Design review of the part built by this model. Coordinates are the model's own, in mm. Face numbers are marked on the shaded views. A direction names the side the tool comes from. Round coordinates to 2 decimals unless told otherwise and drop trailing zeros. Loops run counter-clockwise (first coordinate to the right, second up) from the corner with the lowest first, then second, coordinate; pieces in that order, holes last. Notation, with made-up numbers: (-6, -25.5) - (40, -25.5) arc R23 ccw to (40, -4.5) - close; hole circle Ø1 at (-3, 30). An arc over 180 degrees is marked (long way). Return JSON: item names as keys, results as strings. Group by question number.
(1) Wall thickness on L1, parallel to Y at x = 12, z = 2.5; L2, parallel to Y at x = 0.7, z = 6; L3, parallel to Y at x = 10.75, z = -1.75: over which ranges is each line inside the solid? List them lowest first. Write a range as [from, to].
(2) We need section C-C, the plane z = -10. Write out the cut boundary in (x, y).
(3) For the marked faces 1, 2, 3 and 4, list the 3-axis set-ups (+Z, -Z, +X, -X, +Y, -Y) from which the entire face can be reached by the end or side of a thin tool; tool diameter is ignored.
(4) The part is to be moulded in two halves that separate along Y. For the marked faces 5, 6 and 7, say which applies: pulls with the +Y half, pulls with the -Y half, needs draft (parallel to the pull), parting line crosses it, or undercut.
(5) We need section D-D, the plane z = 6. Write out the cut boundary in (x, y).
(6) We need section A-A, the plane y = 1.5. Write out the cut boundary in (x, z).
(7) We need section B-B, the plane x = 10. Write out the cut boundary in (y, z).
(8) Clearance check with flat-ended pins moving along their axes: pin 1 (10 mm diameter, centred on x = 2.5, z = -1, fed in from -Y); pin 2 (3 mm diameter, centred on y = 2, z = 6, fed in from +X); pin 3 (5 mm diameter, centred on x = 8.5, y = -5, fed in from -Z); pin 4 (8.5 mm diameter, centred on x = 10, z = -10, fed in from -Y). State where each tip first meets the part, or that it passes through.
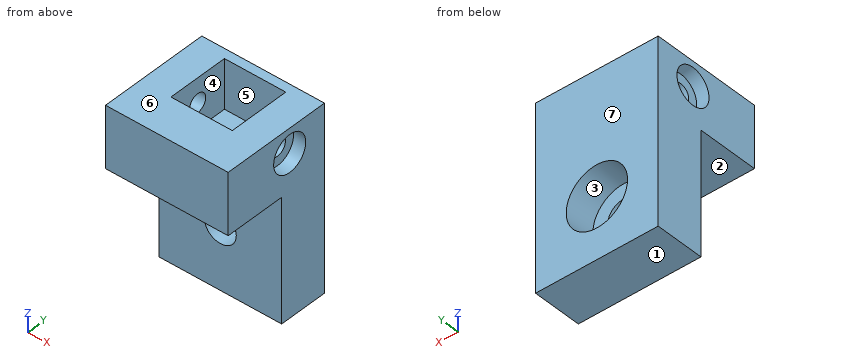
from build123d import *

# Parameters (mm, degrees)
SKETCH_1_W          = 20
SKETCH_1_H          = 20
EXTRUDE_1_DEPTH     = 8
EXTRUDE_2_DEPTH     = 20
SKETCH_3_W          = 4
SKETCH_3_H          = 13
EXTRUDE_3_DEPTH     = 20
CUT_EXTRUDE_1_DEPTH = 5
SKETCH_5_R          = 2.6
CUT_EXTRUDE_2_DEPTH = 13
EXTRUDE_4_DEPTH     = 20
SKETCH_9_W          = 20
SKETCH_9_H          = 13
SKETCH_9_W_2        = 10
SKETCH_9_H_2        = 10
EXTRUDE_5_DEPTH     = 26
SKETCH_10_W         = 10
SKETCH_10_H         = 10
CUT_EXTRUDE_3_DEPTH = 14
SKETCH_13_W         = 20
SKETCH_13_H         = 13
CUT_EXTRUDE_4_DEPTH = 20
SKETCH_14_W         = 5
SKETCH_14_H         = 5
CUT_EXTRUDE_5_DEPTH = 8
CUT_EXTRUDE_6_DEPTH = 20
SKETCH_16_R         = 3
CUT_EXTRUDE_7_DEPTH = 2
CUT_EXTRUDE_START   = -2
SKETCH_17_R         = 3
CUT_EXTRUDE_8_DEPTH = 2
SKETCH_18_W         = 20
SKETCH_18_H         = 4
CUT_EXTRUDE_9_DEPTH = 20
SKETCH_19_W         = 10
SKETCH_19_H         = 5
EXTRUDE_6_DEPTH     = 20


with BuildPart() as part:
    # 草图1 → 凸台-拉伸1 (new body)
    with BuildSketch(Plane(origin=(0, 0, 0), x_dir=(1, 0, 0), z_dir=(0, 1, 0))):
        with Locations((10, 10)):
            Rectangle(SKETCH_1_W, SKETCH_1_H)
    extrude(amount=EXTRUDE_1_DEPTH)

    # 草图2 → 凸台-拉伸2 (add)
    with BuildSketch(Plane.ZY):
        Polygon((-24, 0), (-24, -5), (-20, -5), (-20, 0), (-20, 8), (-24, 8), align=None)
    extrude(amount=-EXTRUDE_2_DEPTH)

    # 草图3 → 凸台-拉伸3 (add)
    with BuildSketch(Plane.ZY):
        with Locations((2, 1.5)):
            Rectangle(SKETCH_3_W, SKETCH_3_H)
    extrude(amount=-EXTRUDE_3_DEPTH)

    # 草图4 → 切除-拉伸1 (cut)
    with BuildSketch(Plane(origin=(0, 8, 0), x_dir=(1, 0, 0), z_dir=(0, 1, 0))):
        with BuildLine():
            ThreePointArc((15, 10), (10, 15), (5, 10))
            Line((5, 10), (15, 10))
        make_face()
        with BuildLine():
            Line((15, 10), (5, 10))
            ThreePointArc((5, 10), (10, 5), (15, 10))
        make_face()
        with BuildLine():
            ThreePointArc((15, 10), (10, 15), (5, 10))
            Line((5, 10), (15, 10))
        make_face()
        with BuildLine():
            Line((15, 10), (5, 10))
            ThreePointArc((5, 10), (10, 5), (15, 10))
        make_face()
    extrude(amount=-CUT_EXTRUDE_1_DEPTH, mode=Mode.SUBTRACT)

    # 草图5 → 切除-拉伸2 (cut)
    with BuildSketch(Plane(origin=(0, 8, 0), x_dir=(1, 0, 0), z_dir=(0, 1, 0))):
        with Locations(Location((10, 10, 0), (0, 0, 270))):
            Circle(SKETCH_5_R)
    extrude(amount=-CUT_EXTRUDE_2_DEPTH, mode=Mode.SUBTRACT)

    # 草图8 → 凸台-拉伸4 (add)
    with BuildSketch(Plane.XY.offset(4)):
        Polygon((10, 6.5), (15, 6.5), (15, 1.5), (15, -3.5), (10, -3.5), (5, -3.5), (5, 1.5), (5, 6.5), align=None)
    extrude(amount=EXTRUDE_4_DEPTH)

    # 草图9 → 凸台-拉伸5 (add)
    with BuildSketch(Plane.XY.offset(4)):
        with Locations((10, 1.5)):
            Rectangle(SKETCH_9_W, SKETCH_9_H)
        with Locations((10, 1.5)):
            Rectangle(SKETCH_9_W_2, SKETCH_9_H_2, mode=Mode.SUBTRACT)
    extrude(amount=EXTRUDE_5_DEPTH)

    # 草图10 → 切除-拉伸3 (cut)
    with BuildSketch(Plane.XY.offset(24)):
        with Locations((10, 1.5)):
            Rectangle(SKETCH_10_W, SKETCH_10_H)
    extrude(amount=-CUT_EXTRUDE_3_DEPTH, mode=Mode.SUBTRACT)

    # 草图13 → 切除-拉伸4 (cut)
    with BuildSketch(Plane.ZY):
        with Locations((20, 1.5)):
            Rectangle(SKETCH_13_W, SKETCH_13_H)
    extrude(amount=-CUT_EXTRUDE_4_DEPTH, mode=Mode.SUBTRACT)

    # 草图14 → 切除-拉伸5 (cut)
    with BuildSketch(Plane.XY.offset(10)):
        with Locations((7.5, 4)):
            Rectangle(SKETCH_14_W, SKETCH_14_H)
        with Locations((12.5, 4)):
            Rectangle(SKETCH_14_W, SKETCH_14_H)
        with Locations((7.5, -1)):
            Rectangle(SKETCH_14_W, SKETCH_14_H)
        with Locations((12.5, -1)):
            Rectangle(SKETCH_14_W, SKETCH_14_H)
    extrude(amount=-CUT_EXTRUDE_5_DEPTH, mode=Mode.SUBTRACT)

    # 草图15 → 切除-拉伸6 (cut)
    with BuildSketch(Plane.ZY):
        with BuildLine():
            ThreePointArc((4.5, 1.5), (6, 0), (7.5, 1.5))
            Line((7.5, 1.5), (4.5, 1.5))
        make_face()
        with BuildLine():
            Line((4.5, 1.5), (7.5, 1.5))
            ThreePointArc((7.5, 1.5), (6, 3), (4.5, 1.5))
        make_face()
        with BuildLine():
            ThreePointArc((4.5, 1.5), (6, 0), (7.5, 1.5))
            Line((7.5, 1.5), (4.5, 1.5))
        make_face()
        with BuildLine():
            Line((4.5, 1.5), (7.5, 1.5))
            ThreePointArc((7.5, 1.5), (6, 3), (4.5, 1.5))
        make_face()
    extrude(amount=-CUT_EXTRUDE_6_DEPTH, mode=Mode.SUBTRACT)

    # 草图16 → 切除-拉伸7 (cut)
    with BuildSketch(Plane.ZY):
        with Locations((6, 1.5)):
            Circle(SKETCH_16_R)
    extrude(amount=-CUT_EXTRUDE_7_DEPTH, mode=Mode.SUBTRACT)

    # 草图17 → 切除-拉伸8 (cut)
    with BuildSketch(Plane(origin=(20, 0, 0), x_dir=(0, 0, -1), z_dir=(1, 0, 0)).offset(CUT_EXTRUDE_START)):
        with Locations(Location((-6, 1.5, 0), (0, 0, 180))):
            Circle(SKETCH_17_R)
    extrude(amount=CUT_EXTRUDE_8_DEPTH, mode=Mode.SUBTRACT)

    # 草图18 → 切除-拉伸9 (cut)
    with BuildSketch(Plane.XZ.offset(5)):
        with Locations((10, -22)):
            Rectangle(SKETCH_18_W, SKETCH_18_H)
    extrude(amount=-CUT_EXTRUDE_9_DEPTH, mode=Mode.SUBTRACT)

    # 草图19 → 凸台-拉伸6 (add)
    with BuildSketch(Plane(origin=(20, 0, 0), x_dir=(0, 0, -1), z_dir=(1, 0, 0))):
        with Locations((-5, -7.5)):
            Rectangle(SKETCH_19_W, SKETCH_19_H)
    extrude(amount=-EXTRUDE_6_DEPTH)


solid = part.part
Solutions:
{
 "1": {"L1": "[-10, -3.5], [6.5, 8]", "L2": "[-10, -1.5], [4.5, 8]", "L3": "[0, 8]"},
 "2": {"outline": "(0, 0) - (7.4, 0) - (7.4, 3) - (5, 3) - (5, 8) - (0, 8) - close; (12.6, 0) - (20, 0) - (20, 8) - (15, 8) - (15, 3) - (12.6, 3) - close"},
 "3": {"face 1": "-Z, +X, -X, +Y, -Y", "face 2": "-Z, +X, -X, -Y", "face 3": "+Y", "face 4": "+Z"},
 "4": {"face 5": "undercut", "face 6": "needs draft", "face 7": "pulls with the +Y half"},
 "5": {"outline": "(0, -10) - (20, -10) - (20, -1.5) - (18, -1.5) - (18, 0) - (15, 0) - (15, -3.5) - (5, -3.5) - (5, 0) - (2, 0) - (2, -1.5) - (0, -1.5) - close; (0, 4.5) - (2, 4.5) - (2, 3) - (5, 3) - (5, 6.5) - (15, 6.5) - (15, 3) - (18, 3) - (18, 4.5) - (20, 4.5) - (20, 8) - (0, 8) - close"},
 "6": {"outline": "(0, -20) - (20, -20) - (20, 3) - (18, 3) - (18, 4.5) - (15, 4.5) - (15, 2) - (5, 2) - (5, 4.5) - (2, 4.5) - (2, 3) - (0, 3) - close; (0, 9) - (2, 9) - (2, 7.5) - (5, 7.5) - (5, 10) - (0, 10) - close; (15, 7.5) - (18, 7.5) - (18, 9) - (20, 9) - (20, 10) - (15, 10) - close; hole circle Ø5.2 at (10, -10)"},
 "7": {"outline": "(-10, 0) - (0, 0) - (0, -7.4) - (3, -7.4) - (3, -5) - (8, -5) - (8, 10) - (6.5, 10) - (6.5, 2) - (-3.5, 2) - (-3.5, 10) - (-10, 10) - close; (0, -20) - (8, -20) - (8, -15) - (3, -15) - (3, -12.6) - (0, -12.6) - close"},
 "8": {"pin 1": "y = -10", "pin 2": "x = 18", "pin 3": "z = 0", "pin 4": "y = 0"}
}
